Geometry check sheet. Reference: the model listing, model coordinates, mm. A direction names the side the tool comes from. Round coordinates to 2 decimals unless told otherwise and drop trailing zeros. Order: outer loops, then holes, each group sorted by start corner. A loop starts at its lowest first (then second) coordinate and runs counter-clockwise, first axis right, second up. Notation, with made-up numbers: (38, -7.5) - (48, -7.5) arc R25 cw to (48, 14.5) - close; hole circle Ø5 at (20.5, -23.75). An arc over 180 degrees is marked (long way). Return JSON: item names as keys, results as strings. Group by question number.
Q1. Sectioned sample at B-B, the plane x = 0. Record the cut outline in (y, z).
Q2. Tool access check on faces 3 (the flat face through (9, 1, 12)), 4 (the cylindrical face through (-32, 0, 10)). Record the directions out of +Z, -Z, +X, -X, +Y, -Y that give a thin tool (end or side, any length) a straight path to the whole face; none if there is none.
Q3. Gauge pin test, flat ends, axial feed: pin 1 Ø2 at (x, z) = (17.5, 1.5) entering from -Y; pin 2 Ø1 at (x, z) = (28.5, 2.5) entering from -Y; pin 3 Ø7 at (x, y) = (2, -26) entering from +Z. Record the tip position at first contact, or that the pin passes through.
Q4. Material ranges on line 1 along Y through (x, z) = (0, 10.55); line 2 along Y through (x, z) = (17, 8.5); line 3 along Y through (x, z) = (12, 7.75), recorded low to high.
Q5. Draft check along X on faces 1 (the flat face through (-1, 1, 0)), 2 (the flat face through (18, -18, 5)). Enter one of: pulls with the +X half, pulls with the -X half, needs draft (parallel to the pull), parting line crosses it, or undercut.
Q6. Sectioned sample at A-A, the plane y = 0. Record the cut outline in (x, z), then the cut area to 3 significant figures.
Autodesk Inventor part; units mm, degrees
ref_plane "YZ Plane" through (0, 0, 0) normal (1, 0, 0) x (0, 1, 0)
ref_plane "XZ Plane" through (0, 0, 0) normal (0, 1, 0) x (-1, 0, 0)
ref_plane "XY Plane" through (0, 0, 0) normal (0, 0, 1) x (1, 0, 0)
sketch "Sketch1" plane through (0, 0, 0) normal (0, 0, 1) x (1, 0, 0)
  circle A0 centre (0, 0) radius 43
  circle A1 centre (0, 0) radius 7
  circle A2 centre (0, 25) radius 7
  circle A3 centre (-17.6777, 17.6777) radius 7
  circle A4 centre (-25, 0) radius 7
  circle A5 centre (-17.6777, -17.6777) radius 7
  circle A6 centre (0, -25) radius 7
  circle A7 centre (17.6777, -17.6777) radius 7
  circle A8 centre (25, 0) radius 7
  circle A9 centre (17.6777, 17.6777) radius 7
  dimension "diameter" = 14
  dimension "d2" = 14
  dimension "d5" = 360
  dimension "d7" = 25
  dimension "d28" = 86
extrude "Extrusion1" add sketch "Sketch1" along normal blind 12
extrude "Extrusion2" add sketch "Sketch1" along normal blind 2 contours A2
extrude "Extrusion3" add sketch "Sketch1" along normal blind 3 contours A9
extrude "Extrusion4" add sketch "Sketch1" along normal blind 4 contours A8
extrude "Extrusion5" add sketch "Sketch1" along normal blind 5 contours A7
extrude "Extrusion6" add sketch "Sketch1" along normal blind 6 contours A6
extrude "Extrusion7" add sketch "Sketch1" along normal blind 7 contours A5
extrude "Extrusion8" add sketch "Sketch1" along normal blind 8 contours A4
extrude "Extrusion9" add sketch "Sketch1" along normal blind 9 contours A3
extrude "Extrusion10" add sketch "Sketch1" along normal blind 10 contours A1
sketch "Sketch2" plane through (0, 0, 12) normal (0, 0, 1) x (1, 0, 0)
  line L0 (-5.8774, 39.105) -> (5.7366, 39.105) construction
  line L1 (5.7366, 39.105) -> (5.7366, 35.936) construction
  line L2 (5.7366, 35.936) -> (-5.8774, 35.936) construction
  line L3 (-5.8774, 35.936) -> (-5.8774, 39.105) construction
  point P0 (0, 0)
emboss "Emboss1" [suppressed]
chamfer "Chamfer1" distance 1 angle 45 1 edges at (-43, 0, 12)
equation "\"d2\" = diameter"
properties part number "Diameter_14mm"
Reply:
{
 "1": {"outline": "(-43, 0) - (43, 0) - (43, 11) - (42, 12) - (32, 12) - (32, 2) - (18, 2) - (18, 12) - (7, 12) - (7, 10) - (-7, 10) - (-7, 12) - (-18, 12) - (-18, 6) - (-32, 6) - (-32, 12) - (-42, 12) - (-43, 11) - close"},
 "2": {"face 3": "+Z, +X, -X, +Y, -Y", "face 4": "+Z"},
 "3": {"pin 1": "y = -39.71", "pin 2": "y = -32.63", "pin 3": "z = 6"},
 "4": {"line 1": "-43 to -32, -18 to -7, 7 to 18, 32 to 43", "line 2": "-39.5 to -24.64, -10.71 to 10.71, 24.64 to 39.5", "line 3": "-41.29 to -21.77, -13.58 to 13.58, 21.77 to 41.29"},
 "5": {"face 1": "needs draft", "face 2": "undercut"},
 "6": {"outline": "(-43, 0) - (43, 0) - (43, 11) - (42, 12) - (32, 12) - (32, 4) - (18, 4) - (18, 12) - (7, 12) - (7, 10) - (-7, 10) - (-7, 12) - (-18, 12) - (-18, 8) - (-32, 8) - (-32, 12) - (-42, 12) - (-43, 11) - close", "area": "835 mm^2"}
}
